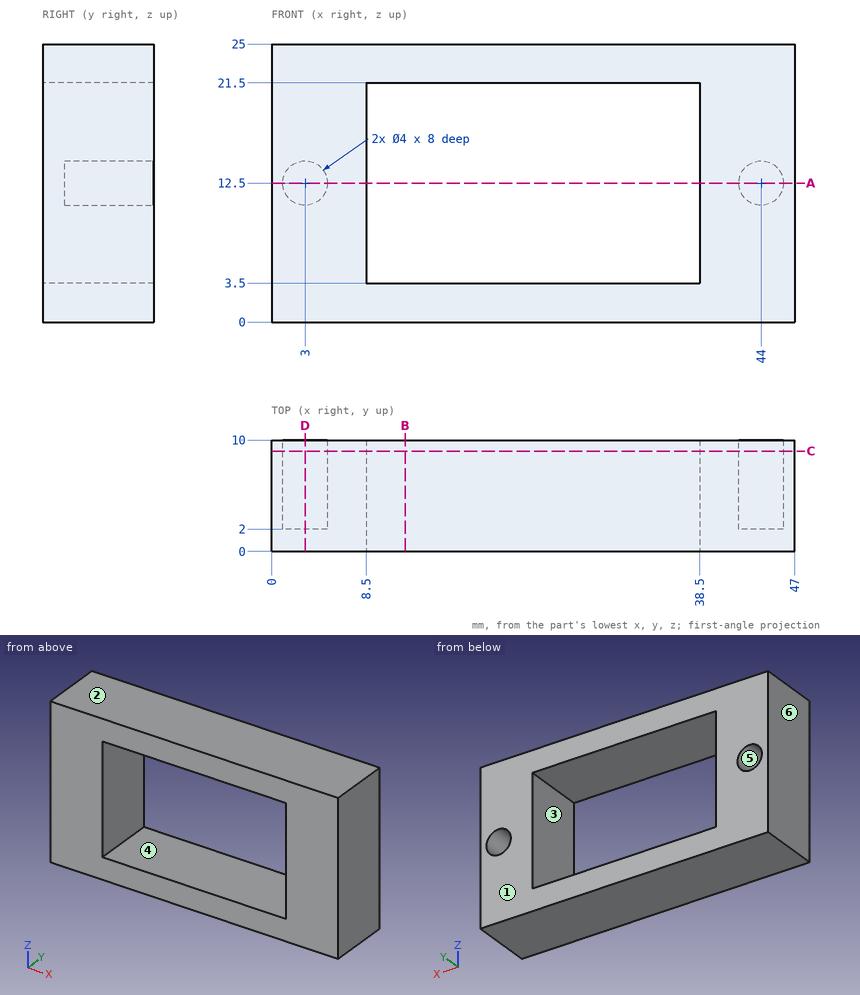
The drawing under review shows one solid part. Ordinate dimensions are in mm from its lowest x, y, z. A direction names the side the tool comes from. Round coordinates to 2 decimals unless told otherwise and drop trailing zeros. Order: outer loops, then holes, each group sorted by start corner. A loop starts at its lowest first (then second) coordinate and runs counter-clockwise, first axis right, second up. Notation, with made-up numbers: (-16, 36.25) - (9, 36.25) arc R9 cw to (9, 49.25) - close; hole circle Ø7 at (18.25, -4.75). An arc over 180 degrees is marked (long way). Return JSON: item names as keys, results as strings.
Q1. Consider section C-C on y = 9. Write out the cut boundary in (x, z), plus the area to 3 significant figures.
Computed values:
{"outline": "(0, 0) - (47, 0) - (47, 25) - (0, 25) - close; hole circle Ø4 at (3, 12.5); hole (8.5, 3.5) - (38.5, 3.5) - (38.5, 21.5) - (8.5, 21.5) - close; hole circle Ø4 at (44, 12.5)", "area": "610 mm2"}
Q2. Machinability: for the marked faces 4, 5 and 6, which of the approach directions +Z, -Z, +X, -X, +Y, -Y give a long, thin tool a straight path to every point of the face, cutting with its end or side? Answer none if there is none.
Computed values:
{"face 4": "+Y, -Y", "face 5": "+Y", "face 6": "+Z, -Z, -X, +Y, -Y"}
Q3. Consider section B-B on x = 12. Write out the cut boundary in (y, z), plus the area to 3 significant figures.
Computed values:
{"outline": "(0, 0) - (10, 0) - (10, 3.5) - (0, 3.5) - close; (0, 21.5) - (10, 21.5) - (10, 25) - (0, 25) - close", "area": "70.0 mm2"}
Q4. The part is to be moulded in two halves that separate along Z. For the marked faces 1, 2 and 3, say which applies: pulls with the +Z half, pulls with the -Z half, needs draft (parallel to the pull), parting line crosses it, or undercut.
Computed values:
{"face 1": "needs draft", "face 2": "pulls with the +Z half", "face 3": "undercut"}
Q5. For pin 1 Ø1.2 at (x, z) = (44, 12) entering from +Y, flat-tipped, find the tip position at first contact; note if it passes through.
Computed values:
{"pin 1": "stops at y = 2"}
Q6. Consider section D-D on x = 3. Write out the cut boundary in (y, z), plus the area to 3 significant figures.
Computed values:
{"outline": "(0, 0) - (10, 0) - (10, 10.5) - (2, 10.5) - (2, 14.5) - (10, 14.5) - (10, 25) - (0, 25) - close", "area": "218 mm2"}
Q7. Consider section A-A on z = 12.5. Write out the cut boundary in (x, y), plus the area to 3 significant figures.
Computed values:
{"outline": "(0, 0) - (8.5, 0) - (8.5, 10) - (5, 10) - (5, 2) - (1, 2) - (1, 10) - (0, 10) - close; (38.5, 0) - (47, 0) - (47, 10) - (46, 10) - (46, 2) - (42, 2) - (42, 10) - (38.5, 10) - close", "area": "106 mm2"}
Q8. Wall thickness on L1, parallel to X at y = 6.5, z = 12.5; L2, parallel to Z at x = 36, y = 1; L3, parallel to Z at x = 44, y = 5.75: over which ranges is each line inside the solid? List them lowest first. Write a range as [from, to].
Computed values:
{"L1": "x = [0, 1], [5, 8.5], [38.5, 42], [46, 47]", "L2": "z = [0, 3.5], [21.5, 25]", "L3": "z = [0, 10.5], [14.5, 25]"}
